Model file for the job. Use its own axes, mm. Face numbers are marked on the shaded views. A direction names the side the tool comes from. Round coordinates to 2 decimals unless told otherwise and drop trailing zeros. Order: outer loops, then holes, each group sorted by start corner. A loop starts at its lowest first (then second) coordinate and runs counter-clockwise, first axis right, second up. Notation, with made-up numbers: (84.5, 63) - (125.5, 63) arc R15 cw to (125.5, 81) - close; hole circle Ø2 at (-37, 75). An arc over 180 degrees is marked (long way). Write item = value, one per line.
```python
from build123d import *

# Parameters (mm, degrees)
SKETCH_1_R             = 10
EXTRUDE_1_DEPTH        = 175
SKETCH_2_W             = 7.534980856
SKETCH_2_H             = 25.851722938
CUT_EXTRUDE_1_DEPTH    = 15
HOLE_WIZARD_M8_1_D     = 6.8
HOLE_WIZARD_M8_1_DEPTH = 12
HOLE_WIZARD_M8_1_TIP   = 2.042926105
CHAMFER_1_SIZE         = 0.5
CHAMFER_4_SIZE         = 0.2
CHAMFER_5_SIZE         = 0.5
CHAMFER_2_SIZE         = 0.5


with BuildPart() as part:
    # 스케치1 → 보스-돌출1 (new body)
    with BuildSketch(Plane(origin=(0, 0, 0), x_dir=(1, 0, 0), z_dir=(0, 1, 0))):
        with Locations(Location((0, 0, 0), (0, 0, 270))):
            Circle(SKETCH_1_R)
    extrude(amount=EXTRUDE_1_DEPTH)

    # 스케치2 → 컷-돌출1 (cut)
    with BuildSketch(Plane(origin=(0, 175, 0), x_dir=(1, 0, 0), z_dir=(0, 1, 0))):
        with Locations((-10.767490428, 0.520710059)):
            Rectangle(SKETCH_2_W, SKETCH_2_H)
        with Locations((10.767490428, 0.520710059)):
            Rectangle(SKETCH_2_W, SKETCH_2_H)
    extrude(amount=-CUT_EXTRUDE_1_DEPTH, mode=Mode.SUBTRACT)

    # M8 나사 구멍1
    with Locations(Plane(origin=(0, 0, 0), x_dir=(-1, 0, 0), z_dir=(0, -1, 0))):
        with Locations((0, 0)):
            Hole(HOLE_WIZARD_M8_1_D / 2, depth=HOLE_WIZARD_M8_1_DEPTH)
            with Locations((0, 0, -(HOLE_WIZARD_M8_1_DEPTH + HOLE_WIZARD_M8_1_TIP / 2))):  # 118° drill point
                Cone(0, HOLE_WIZARD_M8_1_D / 2, HOLE_WIZARD_M8_1_TIP, mode=Mode.SUBTRACT)

    # 모따기1
    chamfer_1_edges = [part.edges().sort_by_distance(p)[0] for p in [
        (0, 175, -10),
        (3.780589618, 175, 9.257815193),
        (7, 175, 0),
        (-7, 175, 0),
    ]]
    chamfer(chamfer_1_edges, length=CHAMFER_1_SIZE)

    # 모따기4
    # the kernel refuses this chamfer: 14.141428429, 0.2 mm, written as the material it takes off along each edge
    with BuildSketch(Plane(origin=(-7, 179.872714198, 7.141428429), x_dir=(0.7673746516372044, 0, 0.6411989894133326), z_dir=(0, -1, 0))) as chamfer_4_piece_1:
        with BuildLine():
            Line((1.58509174, 0), (-CHAMFER_4_SIZE * 0.641198989413, -CHAMFER_4_SIZE * 0.767374651637))
            Line((-CHAMFER_4_SIZE * 0.641198989413, -CHAMFER_4_SIZE * 0.767374651637), (0, 0))
            ThreePointArc((0, 0), (1.074309981, 0.027485583), (1.58509174, 0))
        make_face()
    extrude(amount=19.872714198, mode=Mode.SUBTRACT)
    with BuildSketch(Plane(origin=(7, 179.872714198, 7.141428429), x_dir=(-0.7673746516372026, 0, 0.6411989894133348), z_dir=(0, -1, 0))) as chamfer_4_piece_2:
        with BuildLine():
            Line((1.58509174, 0), (-CHAMFER_4_SIZE * 0.641198989413, CHAMFER_4_SIZE * 0.767374651637))
            Line((-CHAMFER_4_SIZE * 0.641198989413, CHAMFER_4_SIZE * 0.767374651637), (0, 0))
            ThreePointArc((0, 0), (1.074309981, -0.027485583), (1.58509174, 0))
        make_face()
    extrude(amount=19.872714198, mode=Mode.SUBTRACT)

    # 모따기5
    # the kernel refuses this chamfer: 35.353571071, 0.5 mm, written as the material it takes off along each edge
    with BuildSketch(Plane(origin=(7, 184.418230147, -7.141428429), x_dir=(-0.7979254789483874, 0, -0.6027561115782952), z_dir=(0, -1, 0))) as chamfer_5_piece_1:
        with BuildLine():
            Line((2.561877444, 0), (-CHAMFER_5_SIZE * 0.602756111578, -CHAMFER_5_SIZE * 0.797925478948))
            Line((-CHAMFER_5_SIZE * 0.602756111578, -CHAMFER_5_SIZE * 0.797925478948), (0, 0))
            ThreePointArc((0, 0), (1.978478429, 0.058021773), (2.561877444, 0))
        make_face()
    extrude(amount=24.418230147, mode=Mode.SUBTRACT)
    with BuildSketch(Plane(origin=(-7, 184.418230147, -7.141428429), x_dir=(0.797925478948387, 0, -0.6027561115782961), z_dir=(0, -1, 0))) as chamfer_5_piece_2:
        with BuildLine():
            Line((2.561877444, 0), (-CHAMFER_5_SIZE * 0.602756111578, CHAMFER_5_SIZE * 0.797925478948))
            Line((-CHAMFER_5_SIZE * 0.602756111578, CHAMFER_5_SIZE * 0.797925478948), (0, 0))
            ThreePointArc((0, 0), (1.978478429, -0.058021773), (2.561877444, 0))
        make_face()
    extrude(amount=24.418230147, mode=Mode.SUBTRACT)

    # 모따기2
    # the kernel refuses this chamfer: 0.5 mm, written as the material it takes off along each edge
    with BuildSketch(Plane(origin=(0, 160, 0), x_dir=(-0.6999999999999962, 0, 0.7141428428542888), z_dir=(0.7141428428542888, 0, 0.6999999999999962))) as chamfer_2_piece_1_section:
        Polygon((10, CHAMFER_2_SIZE), (10 - CHAMFER_2_SIZE, 0), (10, 0), align=None)
    chamfer_2_piece_1 = revolve(axis=Axis((0, 160, 0), (0, -1, 0)), revolution_arc=113.236333046, mode=Mode.PRIVATE)
    chamfer_2_piece_1 = split(chamfer_2_piece_1, bisect_by=Plane(origin=(-7, 160, 0), z_dir=(-1, 0, 0)), keep=Keep.TOP, mode=Mode.PRIVATE)
    add(chamfer_2_piece_1, mode=Mode.SUBTRACT)
    with BuildSketch(Plane(origin=(0, 160, 0), x_dir=(-0.6999999999999962, 0, 0.7141428428542888), z_dir=(0.7141428428542888, 0, 0.6999999999999962))) as chamfer_2_piece_2_section:
        Polygon((10, CHAMFER_2_SIZE), (10 - CHAMFER_2_SIZE, 0), (10, 0), align=None)
    chamfer_2_piece_2 = revolve(axis=Axis((0, 160, 0), (0, -1, 0)), revolution_arc=113.236333046, mode=Mode.PRIVATE)
    chamfer_2_piece_2 = split(chamfer_2_piece_2, bisect_by=Plane(origin=(-6.970714214, 160, 6.970714214), z_dir=(-0.7071067811840911, 0, 0.707106781189004)), keep=Keep.TOP, mode=Mode.PRIVATE)
    add(chamfer_2_piece_2, mode=Mode.SUBTRACT)
    with BuildSketch(Plane(origin=(0, 160, 0), x_dir=(-0.6999999999999962, 0, 0.7141428428542888), z_dir=(0.7141428428542888, 0, 0.6999999999999962))) as chamfer_2_piece_3_section:
        Polygon((10, CHAMFER_2_SIZE), (10 - CHAMFER_2_SIZE, 0), (10, 0), align=None)
    chamfer_2_piece_3 = revolve(axis=Axis((0, 160, 0), (0, -1, 0)), revolution_arc=113.236333046, mode=Mode.PRIVATE)
    chamfer_2_piece_3 = split(chamfer_2_piece_3, bisect_by=Plane(origin=(-6.820714214, 160, -6.820714214), z_dir=(-0.707106781186502, 0, -0.707106781186593)), keep=Keep.TOP, mode=Mode.PRIVATE)
    add(chamfer_2_piece_3, mode=Mode.SUBTRACT)
    with BuildSketch(Plane(origin=(0, 160, 0), x_dir=(0.38004811354694096, 0, -0.9249667190712385), z_dir=(-0.9249667190712385, 0, -0.38004811354694096))) as chamfer_2_piece_4_section:
        Polygon((10, CHAMFER_2_SIZE), (10 - CHAMFER_2_SIZE, 0), (10, 0), align=None)
    chamfer_2_piece_4 = revolve(axis=Axis((0, 160, 0), (0, -1, 0)), revolution_arc=113.236333046, mode=Mode.PRIVATE)
    chamfer_2_piece_4 = split(chamfer_2_piece_4, bisect_by=Plane(origin=(7, 160, 0), z_dir=(1, 0, 0)), keep=Keep.TOP, mode=Mode.PRIVATE)
    add(chamfer_2_piece_4, mode=Mode.SUBTRACT)
    with BuildSketch(Plane(origin=(0, 160, 0), x_dir=(0.38004811354694096, 0, -0.9249667190712385), z_dir=(-0.9249667190712385, 0, -0.38004811354694096))) as chamfer_2_piece_5_section:
        Polygon((10, CHAMFER_2_SIZE), (10 - CHAMFER_2_SIZE, 0), (10, 0), align=None)
    chamfer_2_piece_5 = revolve(axis=Axis((0, 160, 0), (0, -1, 0)), revolution_arc=113.236333046, mode=Mode.PRIVATE)
    chamfer_2_piece_5 = split(chamfer_2_piece_5, bisect_by=Plane(origin=(6.820714214, 160, -6.820714214), z_dir=(0.707106781186502, 0, -0.707106781186593)), keep=Keep.TOP, mode=Mode.PRIVATE)
    add(chamfer_2_piece_5, mode=Mode.SUBTRACT)
    with BuildSketch(Plane(origin=(0, 160, 0), x_dir=(0.38004811354694096, 0, -0.9249667190712385), z_dir=(-0.9249667190712385, 0, -0.38004811354694096))) as chamfer_2_piece_6_section:
        Polygon((10, CHAMFER_2_SIZE), (10 - CHAMFER_2_SIZE, 0), (10, 0), align=None)
    chamfer_2_piece_6 = revolve(axis=Axis((0, 160, 0), (0, -1, 0)), revolution_arc=113.236333046, mode=Mode.PRIVATE)
    chamfer_2_piece_6 = split(chamfer_2_piece_6, bisect_by=Plane(origin=(6.970714214, 160, 6.970714214), z_dir=(0.7071067811840911, 0, 0.707106781189004)), keep=Keep.TOP, mode=Mode.PRIVATE)
    add(chamfer_2_piece_6, mode=Mode.SUBTRACT)
    with BuildSketch(Plane(origin=(0, 160, 0), x_dir=(0.6999999999991152, 0, 0.7141428428551523), z_dir=(0.7141428428551523, 0, -0.6999999999991152))) as chamfer_2_piece_7_section:
        Polygon((10, CHAMFER_2_SIZE), (10 - CHAMFER_2_SIZE, 0), (10, 0), align=None)
    chamfer_2_piece_7 = revolve(axis=Axis((0, 160, 0), (0, -1, 0)), revolution_arc=16.458800605, mode=Mode.PRIVATE)
    chamfer_2_piece_7 = split(chamfer_2_piece_7, bisect_by=Plane(origin=(6.970714214, 160, 6.970714214), z_dir=(0.7071067811840911, 0, 0.707106781189004)), keep=Keep.TOP, mode=Mode.PRIVATE)
    add(chamfer_2_piece_7, mode=Mode.SUBTRACT)
    with BuildSketch(Plane(origin=(0, 160, 0), x_dir=(-0.6999999999991152, 0, 0.7141428428551523), z_dir=(-0.7141428428551523, 0, -0.6999999999991152))) as chamfer_2_piece_8_section:
        Polygon((10, -CHAMFER_2_SIZE), (10 - CHAMFER_2_SIZE, 0), (10, 0), align=None)
    chamfer_2_piece_8 = revolve(axis=Axis((0, 160, 0), (0, 1, 0)), revolution_arc=16.458800605, mode=Mode.PRIVATE)
    chamfer_2_piece_8 = split(chamfer_2_piece_8, bisect_by=Plane(origin=(-6.970714214, 160, 6.970714214), z_dir=(-0.7071067811840911, 0, 0.707106781189004)), keep=Keep.TOP, mode=Mode.PRIVATE)
    add(chamfer_2_piece_8, mode=Mode.SUBTRACT)


solid = part.part
```
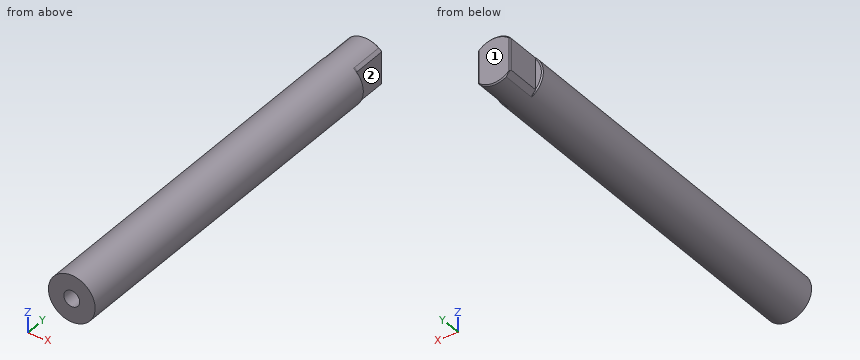
1) Wall check: line 1 along Z through (x, y) = (0, 4); line 2 along X through (y, z) = (118, 7.5); line 3 along Z through (x, y) = (0.25, 46). Give the ranges that are in metal, low to high.
Conclusion:
line_1 = -10 to -3.4, 3.4 to 10
line_2 = -6.61 to 6.61
line_3 = -10 to 10
2) 3-axis set-ups, long thin cutter, end or side, ignore diameter. For the marked faces 1 and 2: which of +Z, -Z, +X, -X, +Y, -Y reach the whole face in a straight line?
Conclusion:
face_1 = +Z, -Z, +X, -X, +Y
face_2 = +Z, -Z, +X, +Y
3) Flat gauge pins, fed straight in: pin 1 Ø7 at (y, z) = (170.5, 0.5) entering from -X; pin 2 Ø0.8 at (x, z) = (-8, -2) entering from +Y; pin 3 Ø2 at (y, z) = (89.5, -6.5) entering from +X. Where does each tip first touch, or does it go through?
Conclusion:
pin_1 = -7
pin_2 = 160
pin_3 = 8.35
4) Cut at A-A (y = 96). Write the cut outline in (x, z), and give its area (3 significant figures).
Conclusion:
outline = circle Ø20 at (0, 0)
area = 314 mm^2
